```python
from build123d import *

# Parameters (mm, degrees)
F0_R     = 20
F1_DEPTH = 10
F2_R     = 12.5
F3_DEPTH = 10
F4_R     = 5
F5_DEPTH = 10


with BuildPart() as f1:
    # F0 (on Top) → F1 (new body)
    with BuildSketch(Plane.XY):
        Circle(F0_R)
    extrude(amount=F1_DEPTH)

    # F2 (on face) → F3 (cut)
    with BuildSketch(Plane.XY.offset(10)):
        Circle(F2_R)
    extrude(amount=-F3_DEPTH, mode=Mode.SUBTRACT)

    # F4 (on face) → F5 (join, through all)
    with BuildSketch(Plane.XY.offset(10)):
        with Locations((0, 20)):
            Circle(F4_R)
    extrude(amount=-F5_DEPTH)


solid = f1.part
```
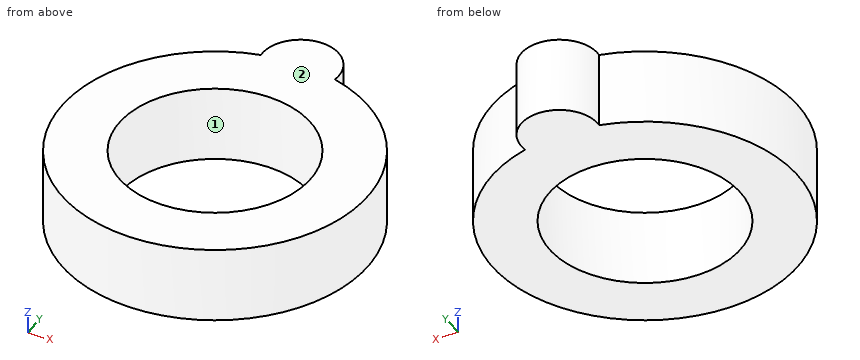
The listing builds one solid part. Answer for the finished solid, in the listing's coordinates (mm). Face numbers are marked on the shaded views. Give positions to 0.01 mm unless a question says otherwise; leave off trailing zeros. Loops run counter-clockwise (first coordinate to the right, second up) from the corner with the lowest first, then second, coordinate; pieces in that order, holes last. Notation, with made-up numbers: M 4,59 L 49,59 A12 cw 49,78 Z; hole C -11,43.25 d6. An arc over 180 degrees is marked long. One line per item, written item: value.
Q1. Determine the mould class of the marked faces 1 and 2 for opening direction Y: +Y half, -Y half, draft (parallel to the pull), parting line (faces both ways), or undercut.
Working result:
face 1: undercut
face 2: draft
Q2. A cutting plane is placed at D-D on y = 20. Determine the outline of the cut face in (x, z).
Working result:
outline: M -5,0 L 5,0 L 5,10 L -5,10 Z
Q3. Find the intervals of material crossed by line 1 (Y direction, x = 0, z = 3.5); line 2 (X direction, y = 20, z = 5); line 3 (X direction, y = 11.5, z = 2.5), in increasing order. Write a range as from..to.
Working result:
line 1: y = -20..-12.5, 12.5..25
line 2: x = -5..5
line 3: x = -16.36..-4.9, 4.9..16.36
Q4. A cutting plane is placed at B-B on y = 0. Determine the outline of the cut face in (x, z).
Working result:
outline: M -20,0 L -12.5,0 L -12.5,10 L -20,10 Z; M 12.5,0 L 20,0 L 20,10 L 12.5,10 Z
Q5. A cutting plane is placed at C-C on z = 5.75. Determine the outline of the cut face in (x, y) (3 decimals), then the cut area to 3 significant figures.
Working result:
outline: M -4.961,19.375 A20 ccw long 4.961,19.375 A5 ccw long Z; hole C 0,0 d25
area: 807 mm^2
Q6. Flat-ended cylindrical pins translate along their axes: P1, Ø4, axis at x = -15.5, z = 9, coming from the -Y side; P2, Ø4, axis at x = -9, y = 0, coming from the +Z side; P3, Ø4, axis at y = -3.5, z = 7.5, coming from the -X side; P4, Ø3, axis at x = -13.5, z = 6, coming from the -Y side. Find the tip coordinate at first contact, or state that the pin passes through.
Working result:
P1: stops at y = -14.76
P2: passes through
P3: stops at x = -19.94
P4: stops at y = -16
Q7. A cutting plane is placed at A-A on x = 0. Determine the outline of the cut face in (y, z).
Working result:
outline: M -20,0 L -12.5,0 L -12.5,10 L -20,10 Z; M 12.5,0 L 25,0 L 25,10 L 12.5,10 Z
